Check sheet for the modelled part. Datum: model origin and axes. Units: mm. Face numbers are marked on the shaded views. A direction names the side the tool comes from. Round coordinates to 2 decimals unless told otherwise and drop trailing zeros. Order: outer loops, then holes, each group sorted by start corner. A loop starts at its lowest first (then second) coordinate and runs counter-clockwise, first axis right, second up. Notation, with made-up numbers: (3.25, 23.25) -> (59.25, 23.25) arc R24 cw to (59.25, 39.25) -> close; hole circle Ø11 at (78, 27.25). An arc over 180 degrees is marked (long way). Answer in a Markdown table with one row per item.
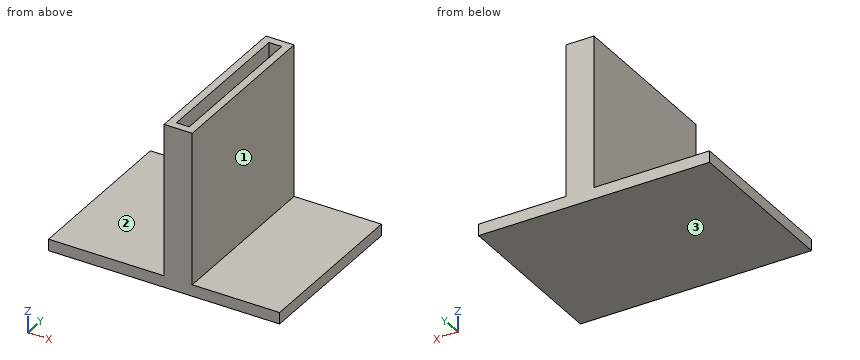
```python
from build123d import *

# Parameters (mm, degrees)
F0_W     = 76.3216018677
F0_H     = 55.6097887456
F1_DEPTH = 3.81
F2_W     = 9.3032829463
F2_H     = 55.6097887456
F3_DEPTH = 50.292
F4_T     = -2.54


with BuildPart() as f1:
    # F0 (on Top) → F1 (new body)
    with BuildSketch(Plane.XY):
        with Locations((38.1608009338, -27.8048943728)):
            Rectangle(F0_W, F0_H)
    extrude(amount=F1_DEPTH)

    # F2 (on face) → F3 (join)
    with BuildSketch(Plane.XY.offset(3.81)):
        with Locations((42.812442407, -27.8048943728)):
            Rectangle(F2_W, F2_H)
    extrude(amount=F3_DEPTH)

    # F4
    f4_openings = [f1.faces().sort_by_distance(p)[0] for p in [
        (42.812442, -27.804894, 54.102),
    ]]
    offset(amount=F4_T, openings=f4_openings, kind=Kind.INTERSECTION)


solid = f1.part
```
(1) Section check A-A on z = 45.5. Record the boundary of the cut face in (x, y).
Solutions:
| item | result |
|---|---|
| outline | (38.16, -55.61) -> (47.46, -55.61) -> (47.46, 0) -> (38.16, 0) -> close; hole (40.7, -53.07) -> (44.92, -53.07) -> (44.92, -2.54) -> (40.7, -2.54) -> close |
(2) Tool access check on the marked faces 1, 2 and 3. Record the directions out of +Z, -Z, +X, -X, +Y, -Y that give a thin tool (end or side, any length) a straight path to the whole face; none if there is none.
Solutions:
| item | result |
|---|---|
| face 1 | +Z, +X, +Y, -Y |
| face 2 | +Z, -X, +Y, -Y |
| face 3 | -Z, +X, -X, +Y, -Y |
(3) Section check B-B on y = -8. Record the boundary of the cut face in (x, z).
Solutions:
| item | result |
|---|---|
| outline | (0, 0) -> (76.32, 0) -> (76.32, 3.81) -> (47.46, 3.81) -> (47.46, 54.1) -> (44.92, 54.1) -> (44.92, 2.54) -> (40.7, 2.54) -> (40.7, 54.1) -> (38.16, 54.1) -> (38.16, 3.81) -> (0, 3.81) -> close |
(4) Section check C-C on x = 5. Record the boundary of the cut face in (y, z), plus the area to 3 significant figures.
Solutions:
| item | result |
|---|---|
| outline | (-55.61, 0) -> (0, 0) -> (0, 3.81) -> (-55.61, 3.81) -> close |
| area | 212 mm^2 |
(5) Scan lines: probe 1 along X at (y, z) = (-22, 37); probe 2 along Y at (x, z) = (41, 13); probe 3 along Z at (x, y) = (37, -7.5). Record each from-to range of solid material in increasing order. Write a range as from..to.
Solutions:
| item | result |
|---|---|
| probe 1 | 38.16..40.7, 44.92..47.46 |
| probe 2 | -55.61..-53.07, -2.54..0 |
| probe 3 | 0..3.81 |
(6) Depth check by flat-ended pin: pin 1 Ø11.5 at (x, y) = (14, -20) entering from +Z; pin 2 Ø25 at (y, z) = (-32.5, 18) entering from -X; pin 3 Ø3 at (y, z) = (-49, 48) entering from +X. Enter the tip coordinate at first touch or a pass-through.
Solutions:
| item | result |
|---|---|
| pin 1 | z = 3.81 |
| pin 2 | x = 38.16 |
| pin 3 | x = 47.46 |
